Source: three-view drawing plus pictorial views. Frame: mm from the lowest corner of the part. A direction names the side the tool comes from. Coordinates: 2 decimals unless noted, no trailing zeros. Write each loop counter-clockwise with the first axis right and the second up, starting at its lowest first coordinate (ties: lowest second). Pieces come first, ordered by that corner, then holes. Notation, with made-up numbers: (9, 45) -> (53, 45) arc R25 cw to (53, 80) -> close; hole circle Ø1 at (78, -2). An arc over 180 degrees is marked (long way). One line per item, written item: value.
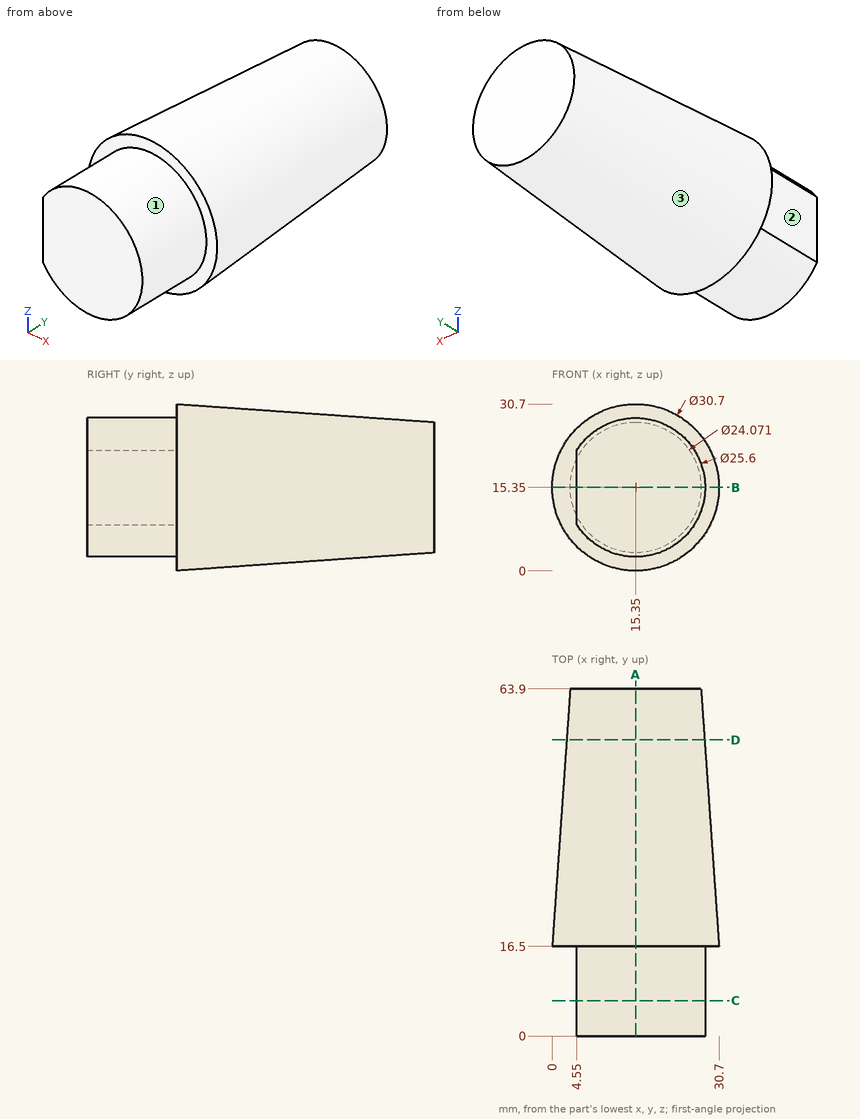
(1) Section B-B (z = 15.35). Return the cut outline in (x, y), then the cut area to 3 significant figures.
Responses:
outline: (0, 16.5) -> (4.55, 16.5) -> (4.55, 0) -> (28.15, 0) -> (28.15, 16.5) -> (30.7, 16.5) -> (27.39, 63.9) -> (3.31, 63.9) -> close
area: 1,690 mm2
(2) Section A-A (x = 15.35). Return the cut outline in (y, z).
Responses:
outline: (0, 2.55) -> (16.5, 2.55) -> (16.5, 0) -> (63.9, 3.31) -> (63.9, 27.39) -> (16.5, 30.7) -> (16.5, 28.15) -> (0, 28.15) -> close
(3) Section D-D (y = 54.5). Return the cut outline in (x, z).
Responses:
outline: circle Ø25.39 at (15.35, 15.35)
(4) Reachability of the marked faces 1, 2 and 3 from +Z, -Z, +X, -X, +Y, -Y: full face, straight path, thin tool, end or side. Return the list, or none.
Responses:
face 1: -Y
face 2: +Z, -Z, -X, -Y
face 3: +Y
(5) Section C-C (y = 6.5). Return the cut outline in (x, z).
Responses:
outline: (4.55, 8.48) arc R12.8 ccw (long way) to (4.55, 22.22) -> close
(6) Line query: line 1 (Z direction, x = 15, y = 13.5); line 2 (Z direction, x = 5, y = 19.5); line 3 (X direction, y = 32, z = 23.5). Output: solid intervals per line, ascending. Write a range as [from, to].
Responses:
line 1: z = [2.55, 28.15]
line 2: z = [4.3, 26.4]
line 3: x = [3.64, 27.06]
(7) First-contact query: pin 1 (1 mm diameter, centred on y = 51, z = 15.5, fed in from -X); pin 2 (6 mm diameter, centred on y = 8.5, z = 3, fed in from +X); pin 3 (2 mm diameter, centred on x = 19, y = 36, fed in from -Z); pin 4 (1.5 mm diameter, centred on x = 27, z = 21, fed in from -Y). Flat tips, straight axial feed; report the tip coordinate or a pass-through.
Responses:
pin 1: stops at x = 2.38
pin 2: stops at x = 24.09
pin 3: stops at z = 1.6
pin 4: stops at y = 0
